Here's how the part is built. I have some questions about the finished solid (model axes, mm). Face numbers are marked on the shaded views. A direction names the side the tool comes from. Round coordinates to 2 decimals unless told otherwise and drop trailing zeros. Loops run counter-clockwise (first coordinate to the right, second up) from the corner with the lowest first, then second, coordinate; pieces in that order, holes last. Notation, with made-up numbers: M 38.5,64 L 77.5,64 A23 ccw 77.5,96 Z; hole C 30,69 d11. An arc over 180 degrees is marked long. Answer as a JSON object with one key per item and string values.
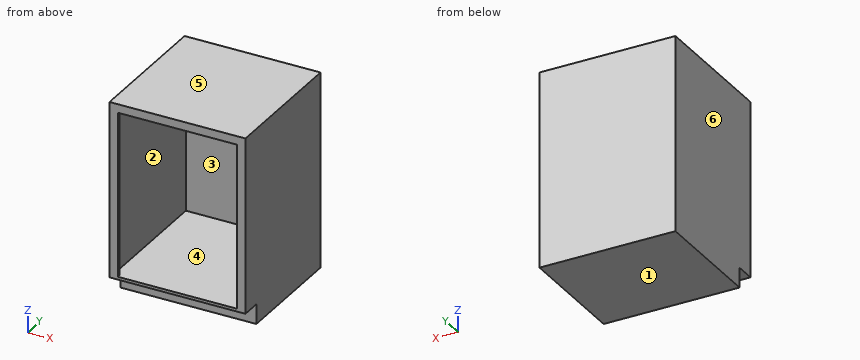
from build123d import *

# Parameters (mm, degrees)
F0_W     = 609.6
F0_H     = 609.6
F1_DEPTH = 876.3
F2_W     = 609.6
F2_H     = 88.9
F3_DEPTH = 88.9
F4_T     = -12.7
F5_DEPTH = 88.9
F6_W     = 609.6
F6_H     = 787.4
F7_DEPTH = 12.7


with BuildPart() as f1:
    # F0 (on Top) → F1 (new body)
    with BuildSketch(Plane.XY):
        with Locations((304.8, -304.8)):
            Rectangle(F0_W, F0_H)
    extrude(amount=F1_DEPTH)

    # F2 (on face) → F3 (cut)
    with BuildSketch(Plane.XZ.offset(609.6)):
        with Locations((304.8, 44.45)):
            Rectangle(F2_W, F2_H)
    extrude(amount=-F3_DEPTH, mode=Mode.SUBTRACT)

    # F4
    f4_openings = [f1.faces().sort_by_distance(p)[0] for p in [
        (304.8, -609.6, 482.6),
    ]]
    offset(amount=F4_T, openings=f4_openings, kind=Kind.INTERSECTION)

    # F5 (add, through all): a face of the model
    f5_faces = [f1.faces().sort_by_distance(p)[0] for p in [
        (304.8, -260.35, 12.7),
    ]]
    extrude(f5_faces, amount=F5_DEPTH)

    # F6 (on face) → F7 (join)
    with BuildSketch(Plane.XZ.offset(609.6)):
        with Locations((304.8, 482.6)):
            Rectangle(F6_W, F6_H)
        Polygon((571.5, 101.6), (38.1, 101.6), (12.7, 101.6), (12.7, 863.6), (596.9, 863.6), (596.9, 101.6), align=None, mode=Mode.SUBTRACT)
        Polygon((38.1, 101.6), (38.1, 838.2), (571.5, 838.2), (571.5, 101.6), (596.9, 101.6), (596.9, 863.6), (12.7, 863.6), (12.7, 101.6), align=None)
    extrude(amount=-F7_DEPTH)


solid = f1.part
Item 1: We'd pull the mould along Z, two halves only. Please class the marked faces 3, 4, 5 and 6: +Z half, -Z half, draft (parallel to the pull), parting line (faces both ways), or undercut.
Solution:
{"face 3": "undercut", "face 4": "undercut", "face 5": "+Z half", "face 6": "draft"}
Item 2: I want a section at A-A on y = -534.5. List the corners of the cut face in (x, z) for me, plus the area to 3 significant figures.
Solution:
{"outline": "M 0,88.9 L 609.6,88.9 L 609.6,876.3 L 0,876.3 Z; hole M 12.7,101.6 L 596.9,101.6 L 596.9,863.6 L 12.7,863.6 Z", "area": "34,800 mm2"}
Item 3: I want a section at C-C on z = 792. List the corners of the cut face in (x, y) for me.
Solution:
{"outline": "M 0,-609.6 L 38.1,-609.6 L 38.1,-596.9 L 12.7,-596.9 L 12.7,-12.7 L 596.9,-12.7 L 596.9,-596.9 L 571.5,-596.9 L 571.5,-609.6 L 609.6,-609.6 L 609.6,0 L 0,0 Z"}
Item 4: For P1, Ø6.5, axis at x = 432, y = -604.5, coming from the -Z side; P2, Ø6, axis at x = 176.5, z = 602.5, coming from the -Y side, each with a flat end and sliding along its axis, tell me the tip position at first contact or that it passes through.
Solution:
{"P1": "stops at z = 88.9", "P2": "stops at y = -12.7"}
Item 5: I want a section at B-B on x = 49.5. List the corners of the cut face in (y, z) for me, plus the area to 3 significant figures.
Solution:
{"outline": "M -609.6,88.9 L -520.7,88.9 L -520.7,0 L 0,0 L 0,876.3 L -609.6,876.3 L -609.6,838.2 L -596.9,838.2 L -596.9,863.6 L -12.7,863.6 L -12.7,101.6 L -609.6,101.6 Z", "area": "71,800 mm2"}
Item 6: For the marked faces 1 and 2, which set-ups out of +Z, -Z, +X, -X, +Y, -Y let a thin tool reach every point of the face, with its end or its side?
Solution:
{"face 1": "-Z, +X, -X, +Y, -Y", "face 2": "none"}
Item 7: I want a section at D-D on y = -433.5. List the corners of the cut face in (x, z) for me.
Solution:
{"outline": "M 0,0 L 609.6,0 L 609.6,876.3 L 0,876.3 Z; hole M 12.7,101.6 L 596.9,101.6 L 596.9,863.6 L 12.7,863.6 Z"}
Item 8: If I drill on L1, parallel to Z at x = 568.5, y = -92; L2, parallel to X at y = -99, z = 553; L3, parallel to Z at x = 145, y = -555, over which ranges is the centre line in solid material (lowest first)? Write a range as from..to.
Solution:
{"L1": "z = 0..101.6, 863.6..876.3", "L2": "x = 0..12.7, 596.9..609.6", "L3": "z = 88.9..101.6, 863.6..876.3"}
